Verification items for the finished model (mm, model axes). Coordinates: 2 decimals unless noted, no trailing zeros. Write each loop counter-clockwise with the first axis right and the second up, starting at its lowest first coordinate (ties: lowest second). Pieces come first, ordered by that corner, then holes. Notation, with made-up numbers: M 32.25,-10.5 L 50.25,-10.5 A16 cw 50.25,18.5 Z; hole C 11.25,10.25 d8. An arc over 180 degrees is marked long. One line per item, written item: value.
```python
from build123d import *

# Parameters (mm, degrees)
SKETCH_1_W                                     = 117
SKETCH_1_H                                     = 84
BOTTOM_LOWER_BASE_PLATE_3MM_DEPTH              = 3
SKETCH_3_R                                     = 3.5
BOTTOM_LOWER_SCREW_6MM_THROUGH_DEPTH           = 3
SKETCH_5_R                                     = 16.5
BOTTOM_LOWER_BATTERY_CLEARANCE_33MM_DEPTH      = 3
SKETCH_9_R                                     = 1.5
BOTTOM_LOWER_BUZZER_SOUND_HOLES_3MM_DEPTH      = 3
SKETCH_10_R                                    = 3
BOTTOM_LOWER_CENTER_RAIL_SCREW_HEADS_6MM_DEPTH = 6
SKETCH_11_W                                    = 117
SKETCH_11_H                                    = 1.5
BOTTOM_LOWER_REAR_EXTENSION_1P5MM_DEPTH        = 3


with BuildPart() as part:
    # Эскиз1 → bottom_lower_base_plate_3mm (new body)
    with BuildSketch(Plane.XY):
        with Locations((53.5, 40)):
            Rectangle(SKETCH_1_W, SKETCH_1_H)
    extrude(amount=BOTTOM_LOWER_BASE_PLATE_3MM_DEPTH)

    # Эскиз3 → bottom_lower_screw_6mm_through (cut)
    with BuildSketch(Plane.XY):
        with Locations(Location((12, 7, 0), (0, 0, 180))):
            Circle(SKETCH_3_R)
        with Locations(Location((95, 7, 0), (0, 0, 180))):
            Circle(SKETCH_3_R)
        with Locations(Location((12, 73, 0), (0, 0, 180))):
            Circle(SKETCH_3_R)
        with Locations(Location((95, 73, 0), (0, 0, 180))):
            Circle(SKETCH_3_R)
    extrude(amount=BOTTOM_LOWER_SCREW_6MM_THROUGH_DEPTH, mode=Mode.SUBTRACT)

    # Эскиз5 → bottom_lower_battery_clearance_33mm (cut)
    with BuildSketch(Plane(origin=(0, 8, 0), x_dir=(1, 0, 0), z_dir=(0, 0, 1))):
        with Locations(Location((58.8, 19.5, 0), (0, 0, 180))):
            Circle(SKETCH_5_R)
    extrude(amount=BOTTOM_LOWER_BATTERY_CLEARANCE_33MM_DEPTH, mode=Mode.SUBTRACT)

    # Эскиз9 → bottom_lower_buzzer_sound_holes_3mm (cut)
    with BuildSketch(Plane(origin=(0, 4, 0), x_dir=(1, 0, 0), z_dir=(0, 0, 1))):
        with Locations(Location((27.4, 9.3, 0), (0, 0, 180))):
            Circle(SKETCH_9_R)
        with Locations(Location((27.4, 14.3, 0), (0, 0, 180))):
            Circle(SKETCH_9_R)
        with Locations(Location((27.4, 19.3, 0), (0, 0, 180))):
            Circle(SKETCH_9_R)
        with Locations(Location((32.4, 9.3, 0), (0, 0, 180))):
            Circle(SKETCH_9_R)
        with Locations(Location((32.4, 14.3, 0), (0, 0, 180))):
            Circle(SKETCH_9_R)
        with Locations(Location((32.4, 19.3, 0), (0, 0, 180))):
            Circle(SKETCH_9_R)
        with Locations(Location((37.4, 9.3, 0), (0, 0, 180))):
            Circle(SKETCH_9_R)
        with Locations(Location((37.4, 14.3, 0), (0, 0, 180))):
            Circle(SKETCH_9_R)
        with Locations(Location((37.4, 19.3, 0), (0, 0, 180))):
            Circle(SKETCH_9_R)
    extrude(amount=BOTTOM_LOWER_BUZZER_SOUND_HOLES_3MM_DEPTH, mode=Mode.SUBTRACT)

    # Эскиз10 → bottom_lower_center_rail_screw_heads_6mm (cut)
    with BuildSketch(Plane.XY):
        with Locations(Location((4, 25, 0), (0, 0, 180))):
            Circle(SKETCH_10_R)
        with Locations(Location((4, 55, 0), (0, 0, 180))):
            Circle(SKETCH_10_R)
        with Locations(Location((103, 25, 0), (0, 0, 180))):
            Circle(SKETCH_10_R)
        with Locations(Location((103, 55, 0), (0, 0, 180))):
            Circle(SKETCH_10_R)
    extrude(amount=BOTTOM_LOWER_CENTER_RAIL_SCREW_HEADS_6MM_DEPTH, mode=Mode.SUBTRACT)

    # Эскиз11 → bottom_lower_rear_extension_1p5mm (add)
    with BuildSketch(Plane.XY):
        with Locations((53.5, 82.75)):
            Rectangle(SKETCH_11_W, SKETCH_11_H)
    extrude(amount=BOTTOM_LOWER_REAR_EXTENSION_1P5MM_DEPTH)


solid = part.part
```
Item 1: Cross-section at D-D, the plane y = 13.3. Enter the section's corners in (x, z), and give its area (3 significant figures).
The answers:
outline: M -5,0 L 25.9,0 L 25.9,3 L -5,3 Z; M 28.9,0 L 30.9,0 L 30.9,3 L 28.9,3 Z; M 33.9,0 L 35.9,0 L 35.9,3 L 33.9,3 Z; M 38.9,0 L 50.4,0 L 50.4,3 L 38.9,3 Z; M 67.2,0 L 112,0 L 112,3 L 67.2,3 Z
area: 274 mm²
Item 2: Cross-section at A-A, the plane x = 95. Enter the section's corners in (y, z), and give its area (4 significant figures).
The answers:
outline: M -2,0 L 3.5,0 L 3.5,3 L -2,3 Z; M 10.5,0 L 69.5,0 L 69.5,3 L 10.5,3 Z; M 76.5,0 L 83.5,0 L 83.5,3 L 76.5,3 Z
area: 214.5 mm²
Item 3: Cross-section at C-C, the plane z = 1.6. Give the number of separate pieces and of enclosed holes in the cut face, and give its area (3 significant figures).
The answers:
separate pieces: 1
enclosed holes: 18
area: 8,820 mm²
Item 4: Cross-section at B-B, the plane x = 58.8. Enter the section's corners in (y, z).
The answers:
outline: M -2,0 L 11,0 L 11,3 L -2,3 Z; M 44,0 L 83.5,0 L 83.5,3 L 44,3 Z
Item 5: Draft check along X on faces 1 (the face through (105.21, 52.97, 1.48)), 2 (the face through (-5, 40, 1)), 3 (the face through (53, 83.5, 1)). Enter one of: released by +X, released by -X, zero draft, split by the parting line, or undercut.
The answers:
face 1: undercut
face 2: released by -X
face 3: zero draft
Item 6: Scan lines: line 1 (Y direction, x = 32.4, z = 2.15); line 2 (X direction, y = 55, z = 2.25); line 3 (Y direction, x = 4, z = 1.5). Record each from-to range of solid material in increasing order.
The answers:
line 1: y = -2 to 11.8, 14.8 to 16.8, 19.8 to 21.8, 24.8 to 83.5
line 2: x = -5 to 1, 7 to 100, 106 to 112
line 3: y = -2 to 22, 28 to 52, 58 to 83.5
